Model file for the job. Use its own axes, mm. A direction names the side the tool comes from. Coordinates: 2 decimals unless noted, no trailing zeros. Order: outer loops, then holes, each group sorted by start corner. A loop starts at its lowest first (then second) coordinate and runs counter-clockwise, first axis right, second up. Notation, with made-up numbers: (8.25, 7) -> (34.25, 7) arc R21 cw to (34.25, 42) -> close; hole circle Ø3 at (-28.5, 17). An arc over 180 degrees is marked (long way). Return JSON: item names as keys, results as strings. Group by question number.
1) Which spindle directions (+Z, -Z, +X, -X, +Y, -Y) get a long thin tool onto all of the face, cutting with end or side? Do faces 1 (the cylindrical face through (-0.54, 2.44, -3.71)), 2 (the flat face through (2.5, 0, -0.5)). Say none if no direction does.
2) Cut at B-B (z = 0.25). Write the cut outline in (x, y), and give its area (3 significant figures).
3) Flat gauge pins, fed straight in: pin 1 (1.6 mm diameter, centred on x = 0, y = 1, fed in from +Z); pin 2 (2 mm diameter, centred on y = 1, z = -4.5, fed in from -X); pin 3 (1 mm diameter, centred on x = -1, z = -5.5, fed in from +Y). Where does each tip first touch, or does it go through?
4) Probe line 1 (X direction, y = 0, z = -4.75); line 2 (Z direction, x = -0.4, y = 1.1). List the from-to ranges inside material, lowest first.
5) Cut at A-A (x = 0). Write the cut outline in (y, z), and give its area (3 significant figures).
6) Cut at D-D (z = -5.25). Write the cut outline in (x, y), and give its area (3 significant figures).
from build123d import *

# Parameters (mm, degrees)
SKETCH2_W           = 0.4
SKETCH2_H           = 2.939387692
CUT_EXTRUDE1_DEPTH  = 10.890399385
SKETCH3_R           = 0.4
BOSS_EXTRUDE1_DEPTH = 1


with BuildPart() as part:
    # Sketch1 → Revolve1 (revolve)
    with BuildSketch(Plane(origin=(0, 0, 0), x_dir=(1, 0, 0), z_dir=(0, 1, 0))):
        with BuildLine():
            Line((0, 0), (0, 9))
            ThreePointArc((0, 9), (1.767766953, 8.267766953), (2.5, 6.5))
            Line((2.5, 6.5), (2.5, 1))
            Line((2.5, 1), (2.9, 1))
            Line((2.9, 1), (2.9, 0))
            Line((2.9, 0), (0, 0))
        make_face()
    revolve(axis=Axis((0, 0, 0), (0, 0, -1)))

    # Sketch2 → Cut-Extrude1 (cut, through all)
    with BuildSketch(Plane.XY):
        with Locations((2.7, 0)):
            Rectangle(SKETCH2_W, SKETCH2_H)
    extrude(amount=-CUT_EXTRUDE1_DEPTH, mode=Mode.SUBTRACT)

    # Sketch3 → Boss-Extrude1 (add)
    with BuildSketch(Plane.XY):
        with Locations((1.27, 0)):
            Circle(SKETCH3_R)
        with Locations(Location((-1.27, 0, 0), (0, 0, 180))):
            Circle(SKETCH3_R)
    extrude(amount=BOSS_EXTRUDE1_DEPTH)


solid = part.part
Answers below:
{
 "1": {"face 1": "-Z", "face 2": "+Z, -Z, +X, +Y, -Y"},
 "2": {"outline": "circle Ø0.8 at (-1.27, 0); circle Ø0.8 at (1.27, 0)", "area": "1.01 mm^2"},
 "3": {"pin 1": "stops at z = 0", "pin 2": "stops at x = -2.5", "pin 3": "stops at y = 2.45"},
 "4": {"line 1": "x = -2.5 to 2.5", "line 2": "z = -8.71 to 0"},
 "5": {"outline": "(-2.9, -1) -> (-2.5, -1) -> (-2.5, -6.5) arc R2.5 ccw to (2.5, -6.5) -> (2.5, -1) -> (2.9, -1) -> (2.9, 0) -> (-2.9, 0) -> close", "area": "43.1 mm^2"},
 "6": {"outline": "circle Ø5 at (0, 0)", "area": "19.6 mm^2"}
}
